from build123d import *

# Parameters (mm, degrees)
F1_DEPTH     = 18.542
F2_R         = 5.6687062333
F3_DEPTH     = 4.064
F4_R         = 2.5242395044
F5_DEPTH     = 18.543
F8_W         = 21.7736046761
F8_H         = 40.5452698469
F9_DEPTH     = 5.334
F10_T1_DEPTH = 65.8569220358
F10_T3_DEPTH = 65.8569220358
F11_R        = 5.5506303957
F12_DEPTH    = 72.686920908


# Not quite as in the source:
# - a fillet or chamfer that OpenCascade refuses, or shapes differently, is made with other operations: its cross-section is extruded or revolved along the edge and cut away or added


with BuildPart() as f1:
    # F0 (on Top) → F1 (new body)
    with BuildSketch(Plane.XY):
        with BuildLine():
            Line((44.45, 25.4), (-44.45, 25.4))
            ThreePointArc((-44.45, 25.4), (-69.85, 0), (-44.45, -25.4))
            Line((-44.45, -25.4), (44.45, -25.4))
            ThreePointArc((44.45, -25.4), (69.85, 0), (44.45, 25.4))
        make_face()
    extrude(amount=F1_DEPTH)

    # F2 (on face) → F3 (cut)
    with BuildSketch(Plane.XY.offset(18.542)):
        with Locations((-44.45, 0)):
            Circle(F2_R)
        with Locations((44.45, 0)):
            Circle(F2_R)
    extrude(amount=-F3_DEPTH, mode=Mode.SUBTRACT)

    # F4 (on face) → F5 (cut, through all)
    with BuildSketch(Plane.XY.offset(18.542)):
        with Locations((-44.45, 0)):
            Circle(F4_R)
        with Locations((44.45, 0)):
            Circle(F4_R)
    extrude(amount=-F5_DEPTH, mode=Mode.SUBTRACT)

    # F8 (on line) → F9 (join, symmetric)
    with BuildSketch(Plane(origin=(0, 0, 0), x_dir=(-0.7071067812, 0.7071067812, 0), z_dir=(0.7071067812, 0.7071067812, 0))):
        with Locations((0, 20.2726349235)):
            Rectangle(F8_W, F8_H)
    extrude(amount=F9_DEPTH, both=True)

    # F10: fillet of radius 11.0377844072 on 2 edges, made by hand

    # F10_s2 → F10_t1 (cut)
    with BuildSketch(Plane(origin=(-23.2839380798, -23.2839380798, 0), x_dir=(0, 0, 1), z_dir=(0.7071067812, 0.7071067812, 0))):
        with BuildLine():
            ThreePointArc((29.5074854397, 10.8868023381), (37.3123776433, 7.6539101345), (40.5452698469, -0.1509820691))
            Line((40.5452698469, -0.1509820691), (40.5452698469, 10.8868023381))
            Line((40.5452698469, 10.8868023381), (29.5074854397, 10.8868023381))
        make_face()
    extrude(amount=F10_T1_DEPTH, mode=Mode.SUBTRACT)

    # F10_s4 → F10_t3 (cut)
    with BuildSketch(Plane(origin=(23.2839380798, 23.2839380798, 0), x_dir=(0, 0, 1), z_dir=(-0.7071067812, -0.7071067812, 0))):
        with BuildLine():
            ThreePointArc((29.5074854397, 10.8868023381), (37.3123776433, 7.6539101345), (40.5452698469, -0.1509820691))
            Line((40.5452698469, -0.1509820691), (40.5452698469, 10.8868023381))
            Line((40.5452698469, 10.8868023381), (29.5074854397, 10.8868023381))
        make_face()
    extrude(amount=F10_T3_DEPTH, mode=Mode.SUBTRACT)

    # F11 (on face) → F12 (cut, through all)
    with BuildSketch(Plane(origin=(3.7717075708, 3.7717075708, 0), x_dir=(-0.7071067812, 0.7071067812, 0), z_dir=(0.7071067812, 0.7071067812, 0))):
        with Locations((0, 31.5257720649)):
            Circle(F11_R)
    extrude(amount=-F12_DEPTH, mode=Mode.SUBTRACT)


solid = f1.part
Check sheet for the modelled part. Datum: model origin and axes. Units: mm. A direction names the side the tool comes from. Round coordinates to 2 decimals unless told otherwise and drop trailing zeros. Order: outer loops, then holes, each group sorted by start corner. A loop starts at its lowest first (then second) coordinate and runs counter-clockwise, first axis right, second up.
(1) Cross-section at D-D, the plane z = 7.5. Enter the section's corners in (x, y), and give its area (3 significant figures).
(2) Cross-section at B-B, the plane z = 34.5. Enter the section's corners in (x, y).
(3) Scan lines: probe 1 along Y at (x, z) = (-44.45, 4.25); probe 2 along Y at (x, z) = (44, 15); probe 3 along Z at (x, y) = (4, 16). Record each from-to range of solid material in increasing order.
(4) Cross-section at A-A, the plane z = 17. Enter the section's corners in (x, y).
(5) Draft check along X on faces 6 (the cylindrical face through (-69.844, 0.559, 9.141)), 7 (the flat face through (-43.27, -2.44, 14.478)), 8 (the flat face through (3.879, 3.664, 24.808)). Enter one of: pulls with the +X half, pulls with the -X half, needs draft (parallel to the pull), parting line crosses it, or undercut.
(6) Cross-section at C-C, the plane x = -15.5. Enter the section's corners in (y, z).
(7) Go/stop test with flat-tipped pins: P1, Ø7, axis at x = 44.45, y = 0, coming from the +Z side; P2, Ø2, axis at x = -48.5, y = 8, coming from the +Z side; P3, Ø4, axis at y = -3, z = 14, coming from the -X side; P4, Ø3.5, axis at x = -45, y = -0.5, coming from the +Z side. Record where each tip stops, or that it passes through.
(8) Access from +Z, -Z, +X, -X, +Y, -Y to the whole of each face (thin tool, end or side, straight path). Record for faces 1 (the flat face through (-7.645, 7.751, 23.948)), 2 (the flat face through (-3.664, -3.879, 24.808)), 3 (the cylindrical face through (46.78, -0.97, 7.34)), 4 (the flat face through (1, 25.4, 9)), 5 (the flat face through (45.63, -2.44, 14.478)).
Check sheet entries:
1. outline: (-44.45, -25.4) - (44.45, -25.4) arc R25.4 ccw to (44.45, 25.4) - (-44.45, 25.4) arc R25.4 ccw to start; hole circle Ø5.05 at (-44.45, 0); hole circle Ø5.05 at (44.45, 0)
1. area: 6,500 mm2
2. outline: (-10.63, 3.08) - (-7.09, -0.46) - (0.46, 7.09) - (-3.08, 10.63) - close; (-0.46, -7.09) - (3.08, -10.63) - (10.63, -3.08) - (7.09, 0.46) - close
3. probe 1: y = -25.4 to -2.52, 2.52 to 25.4
3. probe 2: y = -25.4 to -5.65, 5.65 to 25.4
3. probe 3: z = 0 to 18.54
4. outline: (-44.45, -25.4) - (44.45, -25.4) arc R25.4 ccw to (44.45, 25.4) - (-44.45, 25.4) arc R25.4 ccw to start; hole circle Ø11.34 at (-44.45, 0); hole circle Ø11.34 at (44.45, 0)
5. face 6: pulls with the -X half
5. face 7: undercut
5. face 8: pulls with the +X half
6. outline: (-25.4, 0) - (25.4, 0) - (25.4, 18.54) - (-25.4, 18.54) - close
7. P1: stops at z = 14.48
7. P2: stops at z = 18.54
7. P3: stops at x = -69.83
7. P4: passes through
8. face 1: +Z, -X, +Y
8. face 2: +Z, -X, -Y
8. face 3: +Z, -Z
8. face 4: +Z, -Z, +X, -X, +Y
8. face 5: +Z
